Input: part model. Units: mm. Frame: model coordinates. Coordinates: 2 decimals unless noted, no trailing zeros. Write each loop counter-clockwise with the first axis right and the second up, starting at its lowest first coordinate (ties: lowest second). Pieces come first, ordered by that corner, then holes. Notation, with made-up numbers: (-24.75, 17) - (15.25, 17) arc R36 ccw to (15.25, 54) - close; hole circle Ø6 at (30, 89). An arc over 180 degrees is marked (long way). One line per question, with ' | ' between items. Start each with the question number.
1) Section query A-A on z = -23. Return loops of the section in (x, y).
2) First-contact query: P1, Ø2.5, axis at x = -101.7, z = 15.27, coming from the +Y side (3 decimals); P2, Ø1.5, axis at x = -48, y = -11, coming from the +Z side; P3, Ø1, axis at x = -94.5, y = -10.5, coming from the +Z side. Flat tips, straight axial feed; report the tip coordinate or a pass-through.
3) Section query B-B on y = -10.65. Give the number of separate pieces and of enclosed holes in the cut face, and give its area (3 significant figures).
4) Draft query along X for faces 1 (the cylindrical face through (-44.371, -11.321, 12.145)), 2 (the cylindrical face through (-73.367, -11.321, 28.972)), 3 (the cylindrical face through (-65.839, -11.321, 37.456)), 4 (the cylindrical face through (-54.4, -11.3, -19.9)). Return one class per face: released by +X, released by -X, zero draft, split by the parting line, or undercut.
5) Section query D-D on z = -7.5. Return loops of the section in (x, y).
6) Line query: line 1 (X direction, y = -10.4, z = 23.5); line 2 (Z direction, x = -39, y = -11.6); line 3 (X direction, y = -10.55, z = 28). Output: solid intervals per line, ascending.
7) Section query C-C on x = -61.5. Return loops of the section in (y, z).
```python
from build123d import *

# Parameters (mm, degrees)
SKETCH_2_R      = 1.5
SKETCH_2_R_2    = 1.518721219
SKETCH_2_R_3    = 1.512738874
EXTRUDE_1_DEPTH = 3


with BuildPart() as part:
    # 草图2 → 凸台-拉伸1 (new body)
    with BuildSketch(Plane(origin=(0, -12.8, 0), x_dir=(1, 0, 0), z_dir=(0, 1, 0))):
        with BuildLine():
            Line((-67.750211529, -36.977031927), (-103.858972682, -19.797438789))
            ThreePointArc((-103.858972682, -19.797438789), (-106.429442956, -16.948260564), (-106.232366674, -13.115990359))
            Line((-106.232366674, -13.115990359), (-89.185537995, 30.475859314))
            ThreePointArc((-89.185537995, 30.475859314), (-86.69601178, 33.160837283), (-83.04433662, 33.429381478))
            Line((-83.04433662, 33.429381478), (-44.860392292, 21.55641016))
            ThreePointArc((-44.860392292, 21.55641016), (-43.151818029, 20.629450998), (-41.925856607, 19.120975645))
            Line((-41.925856607, 19.120975645), (-35.176480428, 6.369645252))
            ThreePointArc((-35.176480428, 6.369645252), (-34.651006031, 3.288347657), (-36.057985487, 0.497124446))
            ThreePointArc((-36.057985487, 0.497124446), (-44.450352857, -12.346252855), (-46.996898287, -27.475670456))
            ThreePointArc((-46.996898287, -27.475670456), (-47.856649261, -30.480890326), (-50.332989366, -32.388312117))
            Line((-50.332989366, -32.388312117), (-63.942022797, -37.178376279))
            ThreePointArc((-63.942022797, -37.178376279), (-65.866066657, -37.455025022), (-67.750211529, -36.977031927))
        make_face()
        with Locations(Location((-65.602078267, -32.461998872, 0), (0, 0, 270))):
            Circle(SKETCH_2_R, mode=Mode.SUBTRACT)
        with Locations(Location((-74.632144377, -28.165732348, 0), (0, 0, 270))):
            Circle(SKETCH_2_R, mode=Mode.SUBTRACT)
        with Locations(Location((-83.662210487, -23.869465823, 0), (0, 0, 270))):
            Circle(SKETCH_2_R, mode=Mode.SUBTRACT)
        with Locations(Location((-92.692276597, -19.573199299, 0), (0, 0, 270))):
            Circle(SKETCH_2_R, mode=Mode.SUBTRACT)
        with Locations(Location((-101.704945463, -15.270017578, 0), (0, 0, 270))):
            Circle(SKETCH_2_R_2, mode=Mode.SUBTRACT)
        with Locations(Location((-84.528930836, 28.654867889, 0), (0, 0, 270))):
            Circle(SKETCH_2_R_3, mode=Mode.SUBTRACT)
        with Locations(Location((-74.992068043, 25.689461869, 0), (0, 0, 270))):
            Circle(SKETCH_2_R, mode=Mode.SUBTRACT)
        with Locations(Location((-65.443040865, 22.720273436, 0), (0, 0, 270))):
            Circle(SKETCH_2_R, mode=Mode.SUBTRACT)
        with Locations(Location((-55.894013686, 19.751085004, 0), (0, 0, 270))):
            Circle(SKETCH_2_R, mode=Mode.SUBTRACT)
        with Locations(Location((-46.344986508, 16.781896571, 0), (0, 0, 270))):
            Circle(SKETCH_2_R, mode=Mode.SUBTRACT)
        with Locations(Location((-38.368045535, 1.711376394, 0), (0, 0, 270))):
            Circle(SKETCH_2_R, mode=Mode.SUBTRACT)
        with Locations(Location((-46.778656436, -11.435757143, 0), (0, 0, 270))):
            Circle(SKETCH_2_R, mode=Mode.SUBTRACT)
        with Locations(Location((-49.517857516, -26.800726176, 0), (0, 0, 270))):
            Circle(SKETCH_2_R, mode=Mode.SUBTRACT)
    extrude(amount=EXTRUDE_1_DEPTH)


solid = part.part
```
Answer key:
1) outline: (-92.11, -12.8) - (-66.92, -12.8) - (-66.92, -9.8) - (-92.11, -9.8) - close; (-63.97, -12.8) - (-49.5, -12.8) - (-49.5, -9.8) - (-63.97, -9.8) - close
2) P1: through | P2: z = 31.48 | P3: z = 24.49
3) separate pieces: 1 | enclosed holes: 13 | area: 3,330 mm²
4) face 1: released by +X | face 2: undercut | face 3: split by the parting line | face 4: undercut
5) outline: (-98.17, -12.8) - (-35.77, -12.8) - (-35.77, -9.8) - (-98.17, -9.8) - close
6) line 1: -96.08 to -85.12, -82.21 to -46.94 | line 2: -13.59 to -3.07, -0.35 to 2.82 | line 3: -86.62 to -76.12, -73.14 to -50.42, -48.62 to -47
7) outline: (-12.8, -26.73) - (-9.8, -26.73) - (-9.8, 36.32) - (-12.8, 36.32) - close
